Can you work these out from the model? Positions are in its coordinate system, mm. A direction names the side the tool comes from. Round coordinates to 2 decimals unless told otherwise and drop trailing zeros. Order: outer loops, then holes, each group sorted by start corner. A loop starts at its lowest first (then second) coordinate and runs counter-clockwise, first axis right, second up. Notation, with made-up numbers: M 59,66.5 L 81,66.5 A23 ccw 81,83.5 Z; hole C 48.5,-9 d8. An arc over 180 degrees is marked long. One line per question, with ' | ' between items.
```python
from build123d import *

# Parameters (mm, degrees)
F0_W     = 73.406
F0_H     = 28.575
F2_DEPTH = 14.224
F4_DEPTH = 7.874
F5_DEPTH = 12.7


# Not quite as in the source:
# - a pattern or mirror of a feature is missing from the dataset's text; its kind, count and spacing are read off the source's solid
# - a feature names something its author has since deleted; it is built from what else it names


with BuildPart() as f2:
    # F0 (on Front) → F2 (new body, symmetric)
    with BuildSketch(Plane.XZ):
        Rectangle(F0_W, F0_H)
    extrude(amount=F2_DEPTH, both=True)

    # F3 (on Front) → F4 (join, symmetric)
    with BuildSketch(Plane.XZ):
        Polygon((-36.703, -14.2875), (-36.703, -42.8625), (67.945, -42.8625), (39.37, -14.2875), align=None)
        with BuildLine():
            Line((-6.477, -23.0505), (17.399, -23.0505))
            ThreePointArc((17.399, -23.0505), (21.3503126933, -24.6871873067), (22.987, -28.6385))
            ThreePointArc((22.987, -28.6385), (21.3503126933, -32.5898126933), (17.399, -34.2265))
            Line((17.399, -34.2265), (-6.477, -34.2265))
            ThreePointArc((-6.477, -34.2265), (-12.065, -28.6385), (-6.477, -23.0505))
        make_face(mode=Mode.SUBTRACT)
        Polygon((-36.703, 14.2875), (36.703, 14.2875), (39.37, 14.2875), (50.419, 25.3365), (32.893, 25.3365), (32.893, 42.8625), (-36.703, 42.8625), align=None)
        with BuildLine():
            ThreePointArc((-6.477, 23.0505), (-12.065, 28.6385), (-6.477, 34.2265))
            Line((-6.477, 34.2265), (17.399, 34.2265))
            ThreePointArc((17.399, 34.2265), (21.3503126933, 32.5898126933), (22.987, 28.6385))
            ThreePointArc((22.987, 28.6385), (21.3503126933, 24.6871873067), (17.399, 23.0505))
            Line((17.399, 23.0505), (-6.477, 23.0505))
        make_face(mode=Mode.SUBTRACT)
        Polygon((32.893, 25.3365), (50.419, 25.3365), (67.945, 42.8625), (32.893, 42.8625), align=None)
    extrude(amount=F4_DEPTH, both=True)

    # F3 (on Front) → F5 (join, symmetric)
    with BuildSketch(Plane.XZ):
        Polygon((32.893, 25.3365), (50.419, 25.3365), (67.945, 42.8625), (32.893, 42.8625), align=None)
    f5 = extrude(amount=F5_DEPTH, both=True)

    # F5_copies: F5 across plane
    add(f5.mirror(Plane(origin=(0, 0, 0), x_dir=(-1, 0, 0), z_dir=(0, 0, -1))))


solid = f2.part
```
(1) If we section it at D-D on z = 36: Please give me the cut outline in (x, y), plus the area to 3 significant figures.
Final values:
outline: M -36.7,-7.87 L 32.89,-7.87 L 32.89,-12.7 L 61.08,-12.7 L 61.08,12.7 L 32.89,12.7 L 32.89,7.87 L -36.7,7.87 Z | area: 1,810 mm^2
(2) Will these pins go through, and if not, where does the flat tip stop? pin 1 Ø14.5 at (x, z) = (26, -35.5) entering from -Y; pin 2 Ø12 at (x, z) = (11, 26) entering from +Y; pin 3 Ø4 at (y, z) = (10, -34) entering from -X; pin 4 Ø3 at (x, z) = (1.5, 25.5) entering from +Y.
Final values:
pin 1: y = -12.7 | pin 2: y = 7.87 | pin 3: x = 32.89 | pin 4: through
(3) If we section it at C-C on x = -23.5: Please give me the cut outline in (y, z), plus the area to 3 significant figures.
Final values:
outline: M -14.22,-14.29 L -7.87,-14.29 L -7.87,-42.86 L 7.87,-42.86 L 7.87,-14.29 L 14.22,-14.29 L 14.22,14.29 L 7.87,14.29 L 7.87,42.86 L -7.87,42.86 L -7.87,14.29 L -14.22,14.29 Z | area: 1,710 mm^2
(4) If we section it at B-B on y = -6: Please give me the cut outline in (x, z) (1 decimal), plus the area to 3 significant figures.
Final values:
outline: M -36.7,-42.9 L 67.9,-42.9 L 39.4,-14.3 L 36.7,-14.3 L 36.7,14.3 L 39.4,14.3 L 67.9,42.9 L -36.7,42.9 Z; hole M -6.5,-34.2 L 17.4,-34.2 A5.6 ccw 17.4,-23.1 L -6.5,-23.1 A5.6 ccw Z; hole M -6.5,23.1 L 17.4,23.1 A5.6 ccw 17.4,34.2 L -6.5,34.2 A5.6 ccw Z | area: 6,530 mm^2
(5) On a 3-axis mill with a long thin cutter (end or side, diameter ignored), from which of +Z, -Z, +X, -X, +Y, -Y can I reach the whole of each face in a straight line? I mean faces 1 (the flat face through (46, -12.7, 34)), 2 (the cylindrical face through (-12.064, 0.11, -28.761)), 3 (the flat face through (42, 10, 25.336)). Say none if no direction works.
Final values:
face 1: +Z, +X, -X, -Y | face 2: +Y, -Y | face 3: +X, -X, +Y
(6) Thinking about a two-plate mould opening in X: for faces 4 (the flat face through (32.893, 10, 34)), 5 (the flat face through (46, -12.7, -34)), 6 (the flat face through (6, 0, -34.226)), 7 (the flat face through (5, 0, -23.05)), which applies, released by +X, released by -X, zero draft, split by the parting line, or undercut?
Final values:
face 4: released by -X | face 5: zero draft | face 6: undercut | face 7: undercut
(7) Please list where these lines run through material, in increasing order: probe 1 along Z at (x, y) = (11, 0); probe 2 along Z at (x, y) = (35.5, -9.5); probe 3 along Y at (x, z) = (41.5, 32). Write a range as [from, to].
Final values:
probe 1: [-42.86, -34.23], [-23.05, 23.05], [34.23, 42.86] | probe 2: [-42.86, -25.34], [-14.29, 14.29], [25.34, 42.86] | probe 3: [-12.7, 12.7]
(8) If we section it at A-A on x = 14.5: Please give me the cut outline in (y, z), plus the area to 3 significant figures.
Final values:
outline: M -14.22,-14.29 L -7.87,-14.29 L -7.87,-23.05 L 7.87,-23.05 L 7.87,-14.29 L 14.22,-14.29 L 14.22,14.29 L 7.87,14.29 L 7.87,23.05 L -7.87,23.05 L -7.87,14.29 L -14.22,14.29 Z; M -7.87,-42.86 L 7.87,-42.86 L 7.87,-34.23 L -7.87,-34.23 Z; M -7.87,34.23 L 7.87,34.23 L 7.87,42.86 L -7.87,42.86 Z | area: 1,360 mm^2
